Can you work these out from the drawing? Everything is in mm from the part's minimum corner. A direction names the side the tool comes from. Round coordinates to 2 decimals unless told otherwise and drop trailing zeros. Loops run counter-clockwise (first coordinate to the right, second up) from the corner with the lowest first, then second, coordinate; pieces in that order, holes last. Notation, with made-up numbers: (11.5, 1) -> (27.5, 1) arc R17 ccw to (27.5, 25) -> close; hole circle Ø1 at (40.5, -33). An arc over 180 degrees is marked (long way). One line per item, written item: value.
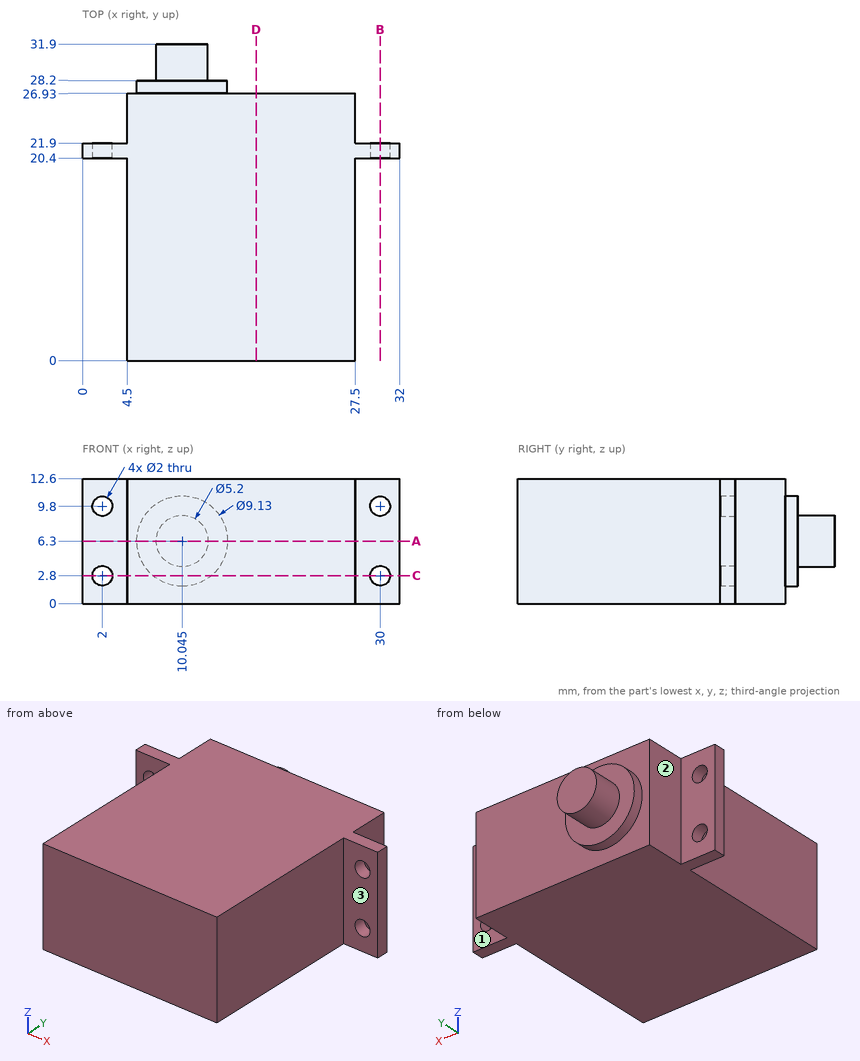
(1) On a 3-axis mill with a long thin cutter (end or side, diameter ignored), from which of +Z, -Z, +X, -X, +Y, -Y can I reach the whole of each face in a straight line? I mean the marked faces 1, 2 and 3. Say none if no direction works.
Results below:
face 1: +Z, -Z, +X, +Y
face 2: +Z, -Z, -X, +Y
face 3: +Z, -Z, +X, -Y
(2) For pin 1 Ø1 at (y, z) = (6, 10.5) entering from +X; pin 2 Ø4 at (y, z) = (15, 4) entering from -X; pin 3 Ø1.3 at (x, z) = (3, 5.5) entering from -Y, each with a flat end and sliding along its axis, tell me the tip position at first contact or that it passes through.
Results below:
pin 1: stops at x = 27.5
pin 2: stops at x = 4.5
pin 3: stops at y = 20.4
(3) Imagine slicing it at D-D on x = 17.5. Write out the boundary of the cut face in (y, z).
Results below:
outline: (0, 0) -> (26.93, 0) -> (26.93, 12.6) -> (0, 12.6) -> close
(4) Imagine slicing it at A-A on z = 6.3. Write out the boundary of the cut face in (x, y) (3 decimals).
Results below:
outline: (0, 20.4) -> (4.5, 20.4) -> (4.5, 0) -> (27.5, 0) -> (27.5, 20.4) -> (32, 20.4) -> (32, 21.9) -> (27.5, 21.9) -> (27.5, 26.93) -> (14.61, 26.93) -> (14.61, 28.2) -> (12.645, 28.2) -> (12.645, 31.9) -> (7.445, 31.9) -> (7.445, 28.2) -> (5.48, 28.2) -> (5.48, 26.93) -> (4.5, 26.93) -> (4.5, 21.9) -> (0, 21.9) -> close
(5) Please list where these lines run through material, in increasing order: L1, parallel to X at y = 21.1, z = 9.8; L2, parallel to X at y = 13.5, z = 10.5; L3, parallel to Y at x = 21.5, z = 11.75.
Results below:
L1: x = 0 to 1, 3 to 29, 31 to 32
L2: x = 4.5 to 27.5
L3: y = 0 to 26.93
(6) Imagine slicing it at B-B on x = 30. Write out the boundary of the cut face in (y, z), then the cut area to 3 significant figures.
Results below:
outline: (20.4, 0) -> (21.9, 0) -> (21.9, 1.8) -> (20.4, 1.8) -> close; (20.4, 3.8) -> (21.9, 3.8) -> (21.9, 8.8) -> (20.4, 8.8) -> close; (20.4, 10.8) -> (21.9, 10.8) -> (21.9, 12.6) -> (20.4, 12.6) -> close
area: 12.9 mm²
(7) Imagine slicing it at C-C on z = 2.8. Write out the boundary of the cut face in (x, y), then the cut area to 3 significant figures.
Results below:
outline: (0, 20.4) -> (1, 20.4) -> (1, 21.9) -> (0, 21.9) -> close; (3, 20.4) -> (4.5, 20.4) -> (4.5, 0) -> (27.5, 0) -> (27.5, 20.4) -> (29, 20.4) -> (29, 21.9) -> (27.5, 21.9) -> (27.5, 26.93) -> (12.98, 26.93) -> (12.98, 28.2) -> (7.11, 28.2) -> (7.11, 26.93) -> (4.5, 26.93) -> (4.5, 21.9) -> (3, 21.9) -> close; (31, 20.4) -> (32, 20.4) -> (32, 21.9) -> (31, 21.9) -> close
area: 634 mm²
